from build123d import *

# Parameters (mm, degrees)
F0_W     = 8.94
F0_H     = 11.46
F0_W_2   = 6.98
F0_H_2   = 7
F1_DEPTH = 3.22
F2_DEPTH = 7.1
F3_R     = 2


with BuildPart() as f1:
    # F0 (on Top) → F1 (new body)
    with BuildSketch(Plane.XY):
        with Locations((4.47, -5.73)):
            Rectangle(F0_W, F0_H)
        with Locations((4.47, -5.6)):
            Rectangle(F0_W_2, F0_H_2, mode=Mode.SUBTRACT)
    extrude(amount=F1_DEPTH)

    # F0 (on Top) → F2 (join)
    with BuildSketch(Plane.XY):
        with Locations((4.47, -5.6)):
            Rectangle(F0_W_2, F0_H_2)
    extrude(amount=F2_DEPTH)

    # F3
    f3_edges = [f1.edges().sort_by_distance(p)[0] for p in [
        (0.98, -9.1, 5.16),
        (7.96, -9.1, 5.16),
        (7.96, -2.1, 5.16),
        (0.98, -2.1, 5.16),
        (8.94, -11.46, 1.61),
        (8.94, 0, 1.61),
        (0, 0, 1.61),
        (0, -11.46, 1.61),
    ]]
    fillet(f3_edges, radius=F3_R)


solid = f1.part
For this review, take the finished solid that the model builds, in its own axes (mm). A direction names the side the tool comes from. Round coordinates to 2 decimals unless told otherwise and drop trailing zeros. Order: outer loops, then holes, each group sorted by start corner. A loop starts at its lowest first (then second) coordinate and runs counter-clockwise, first axis right, second up. Notation, with made-up numbers: (79, -33) -> (114, -33) arc R19 cw to (114, -27) -> close; hole circle Ø9 at (69.25, 19). An arc over 180 degrees is marked (long way). Write item = value, one per line. Start each with the question number.
1) To check wall thickness, follow line 1 (X direction, y = -7, z = 3.75); line 2 (Z direction, x = 2.25, y = -9.75); line 3 (Y direction, x = 3.5, z = 5.25). State the ranges of each line that lie inside material, in increasing order. Write a range as from..to.
2) Take a section at B-B on y = -6.5. State the section outline as (x, z) points, plus the area to 3 significant figures.
3) Tool access review of faces 1 (the face through (7.36, -8.53, 5.19)), 2 (the face through (1.55, -2.7, 5.19)), 3 (the face through (4, -2.1, 5)), 4 (the face through (4, -9.1, 5)): name each direction out of +Z, -Z, +X, -X, +Y, -Y from which nothing blocks a thin tool from reaching the whole face with its end or side.
4) Take a section at C-C on y = -1. State the section outline as (x, z) points, plus the area to 3 significant figures.
5) Insertion check: pin 1 (1.5 mm diameter, centred on x = 5, z = 4.5, fed in from +Y); pin 2 (1.5 mm diameter, centred on x = 8, z = 4, fed in from +Y); pin 3 (1 mm diameter, centred on x = 7, z = 4.5, fed in from -Y). Each pin has a flat end and moves straight along its axis. Give the tip position at first contact, or say it passes through.
6) Take a section at A-A on z = 1.5. State the section outline as (x, y) points.
Verdict:
q1.line_1 = 0.98..7.96
q1.line_2 = 0..3.22
q1.line_3 = -9.1..-2.1
q2.outline = (0, 0) -> (8.94, 0) -> (8.94, 3.22) -> (7.96, 3.22) -> (7.96, 7.1) -> (0.98, 7.1) -> (0.98, 3.22) -> (0, 3.22) -> close
q2.area = 55.9 mm2
q3.face_1 = +Z, +X, -Y
q3.face_2 = +Z, -X, +Y
q3.face_3 = +Z, +X, -X, +Y
q3.face_4 = +Z, +X, -X, -Y
q4.outline = (0.27, 0) -> (8.67, 0) -> (8.67, 3.22) -> (0.27, 3.22) -> close
q4.area = 27.1 mm2
q5.pin_1 = -2.1
q5.pin_2 = -2.57
q5.pin_3 = -9.03
q6.outline = (0, -9.46) arc R2 ccw to (2, -11.46) -> (6.94, -11.46) arc R2 ccw to (8.94, -9.46) -> (8.94, -2) arc R2 ccw to (6.94, 0) -> (2, 0) arc R2 ccw to (0, -2) -> close
